For this review, take the finished solid that the model builds, in its own axes (mm). A direction names the side the tool comes from. Round coordinates to 2 decimals unless told otherwise and drop trailing zeros. Order: outer loops, then holes, each group sorted by start corner. A loop starts at its lowest first (then second) coordinate and runs counter-clockwise, first axis right, second up. Notation, with made-up numbers: (63.25, 56) -> (78.25, 56) arc R20 ccw to (78.25, 71) -> close; hole circle Ø1 at (63.25, 88.5). An arc over 180 degrees is marked (long way). Use a Markdown table: item, result. Add a question column.
1) Clearance check with flat-ended pins moving along their axes: P1, Ø6, axis at x = -641, z = 53.5, coming from the +Y side; P2, Ø5.5, axis at x = -641, y = 220.5, coming from the +Z side; P3, Ø1.5, axis at y = 207, z = 12, coming from the +X side; P4, Ø5.5, axis at x = -657.48, z = 77.57, coming from the +Y side. State where each tip first meets the part, or that it passes through.
2) Consider section C-C (z = 4). State the section outline as (x, y) points (3 decimals), plus the area to 3 significant figures.
3) Consider section B-B (y = 225). State the section outline as (x, z) points, plus the area to 3 significant figures.
4) Machinability: for faces 5 (the face through (-641, 218, 0)), 6 (the face through (-631.01, 219.01, 10.89)), 7 (the face through (-659.2, 202.6, 64.1)), which of the approach directions +Z, -Z, +X, -X, +Y, -Y give a long, thin tool a straight path to every point of the face, cutting with its end or side? Answer none if there is none.
5) Consider section D-D (x = -637). State the section outline as (y, z) points, plus the area to 3 significant figures.
6) Draft analysis for pull direction Y (two halves, no side actions). For faces 1 (the face through (-636, 204.733, 3)), 2 (the face through (-636.519, 227.817, 10.894)), 3 (the face through (-639.71, 202.6, 4.81)), 4 (the face through (-632.952, 207, 11)), state which applies: pulls with the +Y half, pulls with the -Y half, needs draft (parallel to the pull), parting line crosses it, or undercut.
7) Wall thickness on line 1 along Z through (x, y) = (-638.5, 227); line 2 along Y through (x, z) = (-628, 46); line 3 along X through (y, z) = (225, 8): over which ranges is each line inside the solid? List them lowest first. Write a range as [from, to].
8) Consider section A-A (x = -646). State the section outline as (y, z) points, plus the area to 3 significant figures.
```python
from build123d import *

# Parameters (mm, degrees)
SKETCH1_R            = 3.175
BOSS_EXTRUDE1_DEPTH  = 22.098
SKETCH2_W            = 6.364573253
SKETCH2_H            = 22.098
BOSS_EXTRUDE2_DEPTH  = 8.89
SKETCH12_R           = 3.175
BOSS_EXTRUDE6_DEPTH  = 4.326760245
BOSS_EXTRUDE12_DEPTH = 22.098
CUT_EXTRUDE1_DEPTH   = 35.052
BOSS_EXTRUDE13_DEPTH = 22.098
BOSS_EXTRUDE14_REACH = 685.189
SKETCH22_W           = 11.177544577
SKETCH22_H           = 22.098
CUT_EXTRUDE3_DEPTH   = 39.878
CUT_EXTRUDE4_DEPTH   = 684.154025117


with BuildPart() as part:
    # Sketch1 → Boss-Extrude1 (new body)
    with BuildSketch(Plane.XY):
        Polygon((-629.011320926, 228.514758378), (-646.417262265, 232.174381811), (-650.357758597, 213.432549691), (-632.951817258, 209.772926258), align=None)
        with Locations(Location((-635.053635704, 225, 0), (0, 0, 180))):
            Circle(SKETCH1_R, mode=Mode.SUBTRACT)
        with Locations(Location((-637.11116423, 215.213960129, 0), (0, 0, 180))):
            Circle(SKETCH1_R, mode=Mode.SUBTRACT)
    extrude(amount=BOSS_EXTRUDE1_DEPTH)

    # Sketch2 → Boss-Extrude2 (add)
    with BuildSketch(Plane(origin=(15.442364745, 73.44714554, 0), x_dir=(0.9786039871389689, -0.20575285260650125, 0), z_dir=(-0.20575285260650128, -0.978603987138969, 0))):
        with Locations((-677.174764942, 11.049)):
            Rectangle(SKETCH2_W, SKETCH2_H)
    extrude(amount=BOSS_EXTRUDE2_DEPTH)

    # Sketch12 → Boss-Extrude6 (add)
    with BuildSketch(Plane(origin=(0, 204.732760245, 0), x_dir=(1, 0, 0), z_dir=(0, 1, 0))):
        Polygon((-673.909297528, -79.397690297), (-658.291353122, -94.413693096), (-604.598546014, -38.568519939), (-651.343308245, 6.374621247), (-676.077405689, -19.350983895), (-644.950587864, -49.278122283), align=None)
        with Locations(Location((-657.484410814, -77.571736143, 0), (0, 0, 270))):
            Circle(SKETCH12_R, mode=Mode.SUBTRACT)
        with Locations(Location((-616.617520158, -35.066627769, 0), (0, 0, 270))):
            Circle(SKETCH12_R, mode=Mode.SUBTRACT)
    extrude(amount=-BOSS_EXTRUDE6_DEPTH)

    # Sketch19 → Boss-Extrude12 (add)
    with BuildSketch(Plane.XY.offset(22.098)):
        Polygon((-646.417262265, 232.174381811), (-654.037262265, 232.174381811), (-654.037262265, 204.732760245), (-652.186901457, 204.732760245), align=None)
    extrude(amount=-BOSS_EXTRUDE12_DEPTH)

    # Sketch20 → Cut-Extrude1 (cut)
    with BuildSketch(Plane(origin=(0, 0, 0), x_dir=(-1, 0, 0), z_dir=(0, 0, -1))):
        Polygon((629.011320926, 228.514758378), (654.037262265, 232.174381811), (646.417262265, 232.174381811), align=None)
    extrude(amount=-CUT_EXTRUDE1_DEPTH, mode=Mode.SUBTRACT)

    # Sketch21 → Boss-Extrude13 (add)
    with BuildSketch(Plane(origin=(0, 0, 0), x_dir=(-1, 0, 0), z_dir=(0, 0, -1))):
        Polygon((644.129361835, 212.123020588), (644.129361835, 204.732760245), (645.683174376, 204.732760245), align=None)
    extrude(amount=-BOSS_EXTRUDE13_DEPTH)

    # Sketch22 → Boss-Extrude14 (add, up to next)
    with BuildSketch(Plane(origin=(0, 204.732760245, 0), x_dir=(1, 0, 0), z_dir=(0, 1, 0)), mode=Mode.PRIVATE) as boss_extrude14_sk1:
        with Locations((-638.540589547, -11.049)):
            Rectangle(SKETCH22_W, SKETCH22_H)
    boss_extrude14_tool1 = extrude(boss_extrude14_sk1.sketch, amount=BOSS_EXTRUDE14_REACH, mode=Mode.PRIVATE) - part.part
    add(boss_extrude14_tool1.solids().sort_by_distance((-638.54059, 204.73276, 11.049))[0])

    # Sketch23 → Cut-Extrude3 (cut)
    with BuildSketch(Plane.XY.offset(22.098)):
        Polygon((-647.929135227, 231.281170861), (-647.929135227, 204.732760245), (-654.037262265, 204.732760245), (-654.037262265, 232.174381811), align=None)
    extrude(amount=-CUT_EXTRUDE3_DEPTH, mode=Mode.SUBTRACT)

    # Sketch24 → Cut-Extrude4 (cut, through all)
    with BuildSketch(Plane(origin=(0, 204.732760245, 0), x_dir=(1, 0, 0), z_dir=(0, 1, 0))):
        Polygon((-619.246460285, -24.485160698), (-621.00688019, -26.316149982), (-630.161826609, -17.514050456), (-628.401406704, -15.683061172), align=None)
    extrude(amount=-CUT_EXTRUDE4_DEPTH, mode=Mode.SUBTRACT)


solid = part.part
```
Results list:
| question | item | result |
|---|---|---|
| 1 | P1 | y = 204.73 |
| 1 | P2 | z = 22.1 |
| 1 | P3 | x = -632.95 |
| 1 | P4 | through |
| 2 | outline | (-661.318, 200.406) -> (-640.553, 200.406) -> (-640.553, 204.733) -> (-632.952, 204.733) -> (-632.952, 209.773) -> (-629.011, 228.515) -> (-647.929, 231.281) -> (-647.929, 204.733) -> (-661.318, 204.733) -> close; hole circle Ø6.35 at (-637.111, 215.214); hole circle Ø6.35 at (-635.054, 225) |
| 2 | area | 446 mm2 |
| 3 | outline | (-647.93, 0) -> (-638.23, 0) -> (-638.23, 22.1) -> (-647.93, 22.1) -> close; (-631.88, 0) -> (-629.75, 0) -> (-629.75, 22.1) -> (-631.88, 22.1) -> close |
| 3 | area | 261 mm2 |
| 4 | face 5 | -Z, +X, -X, +Y |
| 4 | face 6 | +Z, -Z, +X |
| 4 | face 7 | -X, +Y, -Y |
| 5 | outline | (200.41, 7.42) -> (204.73, 7.42) -> (204.73, 0) -> (212.04, 0) -> (212.04, 22.1) -> (204.73, 22.1) -> (204.73, 72.27) -> (200.41, 72.27) -> close; (218.39, 0) -> (222.49, 0) -> (222.49, 22.1) -> (218.39, 22.1) -> close; (227.51, 0) -> (229.68, 0) -> (229.68, 22.1) -> (227.51, 22.1) -> close |
| 5 | area | 581 mm2 |
| 6 | face 1 | pulls with the -Y half |
| 6 | face 2 | undercut |
| 6 | face 3 | needs draft |
| 6 | face 4 | undercut |
| 7 | line 1 | [0, 22.1] |
| 7 | line 2 | [200.41, 204.73] |
| 7 | line 3 | [-647.93, -638.23], [-631.88, -629.75] |
| 8 | outline | (200.41, -1.24) -> (204.73, -1.24) -> (204.73, 0) -> (231, 0) -> (231, 22.1) -> (204.73, 22.1) -> (204.73, 48.27) -> (200.41, 48.27) -> close; (200.41, 50.37) -> (204.73, 50.37) -> (204.73, 81.63) -> (200.41, 81.63) -> close |
| 8 | area | 930 mm2 |
